The listing builds one solid part. Answer for the finished solid, in the listing's coordinates (mm). A direction names the side the tool comes from. Coordinates: 2 decimals unless noted, no trailing zeros. Order: outer loops, then holes, each group sorted by start corner. A loop starts at its lowest first (then second) coordinate and runs counter-clockwise, first axis right, second up.
```python
from build123d import *

# Parameters (mm, degrees)
SKETCH1_R               = 20.6375
BOSS_EXTRUDE1_DEPTH     = 76.2
SKETCH2_R               = 6.35
CUT_EXTRUDE1_DEPTH      = 38.1
CUT_REVOLVE_THIN1_START = -20.6375
CUT_REVOLVE_THIN1_DEPTH = 14.817629087
SKETCH4_R               = 3.175
CUT_EXTRUDE2_DEPTH      = 6.35


# Read off the part's stored shape, not the designer's step: Cut-Revolve-Thin1
with BuildPart() as part:
    # Sketch1 → Boss-Extrude1 (new body)
    with BuildSketch(Plane(origin=(0, 0, 0), x_dir=(1, 0, 0), z_dir=(0, 1, 0))):
        with Locations(Location((0, 0, 0), (0, 0, 90))):
            Circle(SKETCH1_R)
    extrude(amount=BOSS_EXTRUDE1_DEPTH)

    # Sketch2 → Cut-Extrude1 (cut)
    with BuildSketch(Plane(origin=(0, 76.2, 0), x_dir=(-1, 0, 0), z_dir=(0, 1, 0))):
        with Locations(Location((0, 0, 0), (0, 0, 90))):
            Circle(SKETCH2_R)
    extrude(amount=-CUT_EXTRUDE1_DEPTH, mode=Mode.SUBTRACT)

    # Cut-Revolve-Thin1 outline → Cut-Revolve-Thin1 (cut)
    with BuildSketch(Plane.XY.offset(CUT_REVOLVE_THIN1_START)):
        with BuildLine():
            Line((2.54, 76.2), (-2.54, 76.2))
            ThreePointArc((-2.54, 76.2), (0, 73.66), (2.54, 76.2))
        make_face()
    extrude(amount=CUT_REVOLVE_THIN1_DEPTH, mode=Mode.SUBTRACT)

    # Sketch4 → Cut-Extrude2 (cut)
    with BuildSketch(Plane(origin=(0, 76.2, 0), x_dir=(1, 0, 0), z_dir=(0, 1, 0))):
        with Locations(Location((-13.462, 0, 0), (0, 0, 270))):
            Circle(SKETCH4_R)
        with Locations(Location((13.462, 0, 0), (0, 0, 90))):
            Circle(SKETCH4_R)
    extrude(amount=-CUT_EXTRUDE2_DEPTH, mode=Mode.SUBTRACT)


solid = part.part
```
1) A cutting plane is placed at C-C, the plane x = 0. Write down the section's boundary in (y, z), plus the area to 4 significant figures.
2) Each of these flat-tipped pins is pushed along its axis until it touches: P1, Ø10, axis at y = 9.5, z = -8, coming from the -X side; P2, Ø1, axis at y = 15.5, z = -1.5, coming from the +X side; P3, Ø12, axis at y = 44, z = -13.5, coming from the -X side. Where does it stop, or does it pass through?
3) A cutting plane is placed at D-D, the plane y = 16. Write down the section's boundary in (x, z) (1 decimal).
4) Straight lines are drawn through the part: probe 1 along X at (y, z) = (74, 0); probe 2 along Z at (x, y) = (0, 56). For each, find the intervals that lie inside material, in ascending order.
5) For faces 1 (the cylindrical face through (-0.06, 73.66, -13.33)), 2 (the flat face through (0, 38.1, 0)), 3 (the flat face through (0, 0, 0)), determine the directions among +Z, -Z, +X, -X, +Y, -Y from which every point of the face is accessible in a straight line to the end or side of a thin tool.
6) A cutting plane is placed at A-A, the plane z = 0. Write down the section's boundary in (x, y), plus the area to 3 significant figures.
7) The mould has two halves that part along Z. Classify faces 4 (the cylindrical face through (-20.46, 37.57, 2.69)), 5 (the cylindrical face through (16.56, 73.07, 0.69)), 6 (the flat face through (4.3, 76.2, 4.9)): released by +Z, released by -Z, zero draft, split by the parting line, or undercut.
Working result:
1. outline: (0, -20.64) - (73.66, -20.64) - (73.66, -6.35) - (38.1, -6.35) - (38.1, 6.35) - (76.2, 6.35) - (76.2, 20.64) - (0, 20.64) - close
1. area: 2,625 mm2
2. P1: stops at x = -20.42
2. P2: stops at x = 20.61
2. P3: stops at x = -19.23
3. outline: circle Ø41.3 at (0, 0)
4. probe 1: x = -20.64 to -16.64, -10.29 to -6.35, 6.35 to 10.29, 16.64 to 20.64
4. probe 2: z = -20.64 to -6.35, 6.35 to 20.64
5. face 1: -Z, +Y
5. face 2: +Y
5. face 3: +Z, -Z, +X, -X, -Y
6. outline: (-20.64, 0) - (20.64, 0) - (20.64, 76.2) - (16.64, 76.2) - (16.64, 69.85) - (10.29, 69.85) - (10.29, 76.2) - (6.35, 76.2) - (6.35, 38.1) - (-6.35, 38.1) - (-6.35, 76.2) - (-10.29, 76.2) - (-10.29, 69.85) - (-16.64, 69.85) - (-16.64, 76.2) - (-20.64, 76.2) - close
6. area: 2,580 mm2
7. face 4: split by the parting line
7. face 5: undercut
7. face 6: zero draft
